Part model, mm, in its own coordinate system. Face numbers are marked on the shaded views. Round coordinates to 2 decimals unless told otherwise and drop trailing zeros. Write each loop counter-clockwise with the first axis right and the second up, starting at its lowest first coordinate (ties: lowest second). Pieces come first, ordered by that corner, then holes. Notation, with made-up numbers: (45.25, -16.5) -> (61.25, -16.5) arc R24 ccw to (61.25, 22.5) -> close; hole circle Ø8 at (20.25, -37.75). An arc over 180 degrees is marked (long way). Return JSON: item names as keys, results as strings. Group by question number.
(1) Mould opens along X. For the marked faces 1 and 2 say: +X half, -X half, draft (parallel to the pull), parting line (faces both ways), or undercut.
(2) Drop flat-ended pins along their axis: pin 1 Ø10 at (x, z) = (-25.5, 80) entering from +Y; pin 2 Ø10 at (x, z) = (-45.5, 157) entering from -Y. Give the stop position or say it passes through.
(3) Saw through at C-C (z = -165). List the corners of the cut face in (x, y).
(4) Saw through at B-B (x = -63). List the corners of the cut face in (y, z), plus the area to 3 significant figures.
(5) Saw through at A-A (y = 184). List the corners of the cut face in (x, z).
(6) Drill centre lines: L1, parallel to Z at x = 259.5, y = 8; L2, parallel to Y at x = -73, z = 183.5. Where is each one in solid material? Low to high. Write a range as from..to.
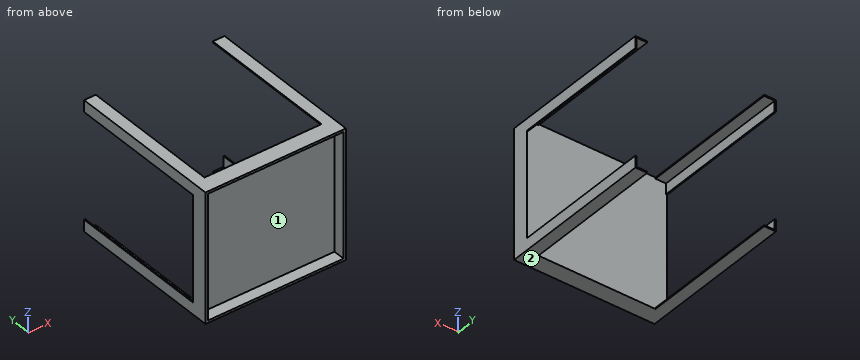
from build123d import *

# Parameters (mm, degrees)
F0_W     = 600
F0_H     = 550
F1_DEPTH = 35
F3_DEPTH = 600
F4_W     = 580
F4_H     = 530
F5_DEPTH = 50


with BuildPart() as f1:
    # F0 (on Front) → F1 (new body, symmetric)
    with BuildSketch(Plane.XZ):
        Rectangle(F0_W, F0_H)
    extrude(amount=F1_DEPTH, both=True)

    # F2 (on face) → F3 (join)
    with BuildSketch(Plane(origin=(0, 35, 0), x_dir=(-1, 0, 0), z_dir=(0, 1, 0))):
        Polygon((250, -275), (300, -275), (300, -225), (295, -225), (295, -270), (250, -270), align=None)
        Polygon((-300, -275), (-250, -275), (-250, -270), (-295, -270), (-295, -225), (-300, -225), align=None)
        Polygon((-250, 270), (-250, 275), (-300, 275), (-300, 225), (-295, 225), (-295, 270), align=None)
        Polygon((295, 225), (300, 225), (300, 275), (250, 275), (250, 270), (295, 270), align=None)
    extrude(amount=F3_DEPTH)

    # F4 (on face) → F5 (cut)
    with BuildSketch(Plane.XZ.offset(35)):
        Rectangle(F4_W, F4_H)
    extrude(amount=-F5_DEPTH, mode=Mode.SUBTRACT)


solid = f1.part
Computed values:
{
 "1": {"face 1": "undercut", "face 2": "draft"},
 "2": {"pin 1": "y = 35", "pin 2": "y = 15"},
 "3": {"outline": "(-300, -35) -> (-290, -35) -> (-290, 15) -> (290, 15) -> (290, -35) -> (300, -35) -> (300, 35) -> (-300, 35) -> close"},
 "4": {"outline": "(-35, -275) -> (35, -275) -> (35, 275) -> (-35, 275) -> (-35, 265) -> (15, 265) -> (15, -265) -> (-35, -265) -> close", "area": "12,000 mm2"},
 "5": {"outline": "(-300, -275) -> (-250, -275) -> (-250, -270) -> (-295, -270) -> (-295, -225) -> (-300, -225) -> close; (-300, 225) -> (-295, 225) -> (-295, 270) -> (-250, 270) -> (-250, 275) -> (-300, 275) -> close; (250, -275) -> (300, -275) -> (300, -225) -> (295, -225) -> (295, -270) -> (250, -270) -> close; (250, 270) -> (295, 270) -> (295, 225) -> (300, 225) -> (300, 275) -> (250, 275) -> close"},
 "6": {"L1": "-275..-265, 265..275", "L2": "15..35"}
}
